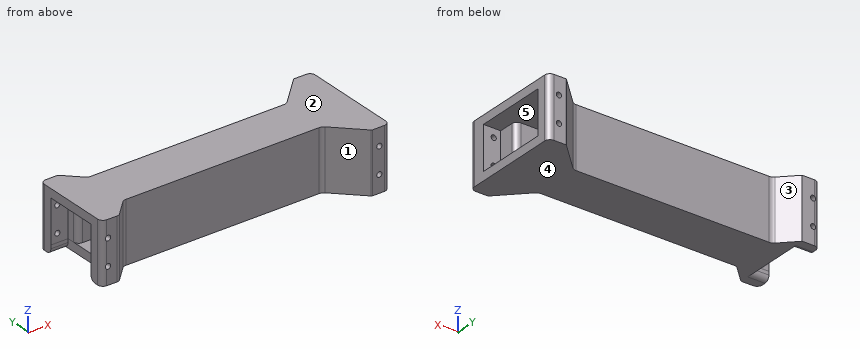
```python
from build123d import *

# Parameters (mm, degrees)
EXTRUDE_1_DEPTH     = 35
SKETCH_2_W          = 25
SKETCH_2_H          = 17
CUT_EXTRUDE_1_DEPTH = 173.018757571
SKETCH_4_W          = 25
SKETCH_4_H          = 13.5
SKETCH_4_H_2        = 11.5
CUT_EXTRUDE_2_DEPTH = 10
SKETCH_7_W          = 25
SKETCH_7_H          = 7
SKETCH_7_H_2        = 6.852029594
CUT_EXTRUDE_5_DEPTH = 10
FILLET_1_R          = 3
SKETCH_9_R          = 1.5
CUT_EXTRUDE_6_DEPTH = 270.810917265
CUT_EXTRUDE_8_DEPTH = 10
FILLET_3_R          = 3


with BuildPart() as part:
    # 草图1 → 凸台-拉伸1 (new body)
    with BuildSketch(Plane.XY):
        with BuildLine():
            Line((107.965790756, 7.914761882), (98.213694846, 7.766808503))
            Line((98.213694846, 7.766808503), (98.92442601, -39.079829993))
            Line((98.92442601, -39.079829993), (108.678766587, -39.079829993))
            ThreePointArc((108.678766587, -39.079829993), (108.959768197, -39.019490003), (109.19628872, -38.856208462))
            Line((109.19628872, -38.856208462), (117.753296763, -30.035556214))
            ThreePointArc((117.753296763, -30.035556214), (118.95311021, -29.207267035), (120.378565842, -28.901176343))
            Line((120.378565842, -28.901176343), (232.012858889, -27.207522891))
            ThreePointArc((232.012858889, -27.207522891), (233.446944009, -27.470230219), (234.671332156, -28.261740759))
            Line((234.671332156, -28.261740759), (250.089839512, -43.21939783))
            ThreePointArc((250.089839512, -43.21939783), (250.331204472, -43.375429159), (250.613907223, -43.427216939))
            Line((250.613907223, -43.427216939), (260.551832391, -43.276444261))
            Line((260.551832391, -43.276444261), (259.64165048, 16.716651749))
            Line((259.64165048, 16.716651749), (249.703725312, 16.565879071))
            ThreePointArc((249.703725312, 16.565879071), (249.422723701, 16.505539082), (249.186203178, 16.34225754))
            Line((249.186203178, 16.34225754), (234.228546108, 0.923750185))
            ThreePointArc((234.228546108, 0.923750185), (233.028732661, 0.095461006), (231.603277029, -0.210629686))
            Line((231.603277029, -0.210629686), (119.968983982, -1.904283139))
            ThreePointArc((119.968983982, -1.904283139), (118.534898862, -1.64157581), (117.310510715, -0.85006527))
            Line((117.310510715, -0.85006527), (108.489858467, 7.706942773))
            ThreePointArc((108.489858467, 7.706942773), (108.248493507, 7.862974102), (107.965790756, 7.914761882))
        make_face()
    extrude(amount=-EXTRUDE_1_DEPTH)

    # 草图2 → 切除-拉伸1 (cut, through all)
    with BuildSketch(Plane(origin=(259.835459196, 3.942079181, 0), x_dir=(0, 0, -1), z_dir=(0.999884933503295, 0.01516969851748372, 0))):
        with Locations((17.5, -17.223957338)):
            Rectangle(SKETCH_2_W, SKETCH_2_H)
    extrude(amount=-CUT_EXTRUDE_1_DEPTH, mode=Mode.SUBTRACT)

    # 草图4 → 切除-拉伸2 (cut)
    with BuildSketch(Plane(origin=(259.835459196, 3.942079181, 0), x_dir=(0, 0, -1), z_dir=(0.999884933503295, 0.01516969851748372, 0))):
        with Locations((17.5, -1.973957338)):
            Rectangle(SKETCH_4_W, SKETCH_4_H)
        with Locations((17.5, -31.473957338)):
            Rectangle(SKETCH_4_W, SKETCH_4_H_2)
    extrude(amount=-CUT_EXTRUDE_2_DEPTH, mode=Mode.SUBTRACT)

    # 草图7 → 切除-拉伸5 (cut)
    with BuildSketch(Plane(origin=(98.308900521, 1.491488003, 0), x_dir=(0, 0, 1), z_dir=(-0.9998849335032951, -0.015169698517482276, 0))):
        with Locations((-17.5, -5.223957338)):
            Rectangle(SKETCH_7_W, SKETCH_7_H)
        with Locations((-17.5, -29.149972135)):
            Rectangle(SKETCH_7_W, SKETCH_7_H_2)
    extrude(amount=-CUT_EXTRUDE_5_DEPTH, mode=Mode.SUBTRACT)

    # 圆角1
    # the kernel refuses this fillet: 3 mm, written as the material it takes off along each edge
    with BuildSketch(Plane(origin=(250.226834538, -21.930615176, -30), x_dir=(0.01516969851748703, -0.9998849335032949, 0), z_dir=(0, 0, 1)), Plane(origin=(249.968949663, -4.932571306, -5), x_dir=(-0.015169698517477554, 0.999884933503295, 0), z_dir=(0, 0, -1))) as fillet_1_piece_1:
        with BuildLine():
            CenterArc((FILLET_1_R, -FILLET_1_R), FILLET_1_R, 90, 90)
            Line((0, -FILLET_1_R), (0, 0))
            Line((0, 0), (FILLET_1_R, 0))
        make_face()
    extrude(amount=25, mode=Mode.SUBTRACT)
    with BuildSketch(Plane(origin=(98.92442601, -39.079829993, 7.387077266), x_dir=(1, 0, 0), z_dir=(0, 0, -1))) as fillet_1_piece_2:
        with BuildLine():
            CenterArc((FILLET_1_R * 0.984943635496, -FILLET_1_R), FILLET_1_R, 90, 89.13080696)
            Line((-FILLET_1_R * 0.0149412980072, -FILLET_1_R * 0.984830301483), (0, 0))
            Line((0, 0), (FILLET_1_R * 0.984943635496, 0))
        make_face()
    extrude(amount=49.774154532, mode=Mode.SUBTRACT)
    with BuildSketch(Plane(origin=(108.678766587, -39.079829993, 3.735844088), x_dir=(0.7926292381316349, 0.6097039370537671, 0), z_dir=(0, 0, -1))) as fillet_1_piece_3:
        with BuildLine():
            CenterArc((1.061212336, -2.968569096), FILLET_1_R, 81.698905724, 45.86919304)
            Line((-0.767899475, -0.590681381), (-0.950810656, -0.35289261))
            Line((-0.950810656, -0.35289261), (-0.182911181, 0.237788771))
            Line((-0.182911181, 0.237788771), (-0.17928295, 0.240536117))
            ThreePointArc((-0.17928295, 0.240536117), (0.589858632, 0.435143228), (1.537650165, 0.29685691))
            Line((1.537650165, 0.29685691), (1.494337635, 0))
        make_face()
    extrude(amount=42.471688176, mode=Mode.SUBTRACT)
    with BuildSketch(Plane(origin=(260.551832391, -43.276444261, 7.5), x_dir=(-0.015169698517487012, 0.9998849335032949, 0), z_dir=(0, 0, -1)), Plane(origin=(98.213694846, 7.766808503, 7.5), x_dir=(0.015169698517482278, -0.999884933503295, 0), z_dir=(0, 0, -1))) as fillet_1_piece_4:
        with BuildLine():
            CenterArc((FILLET_1_R, -FILLET_1_R), FILLET_1_R, 90, 90)
            Line((0, -FILLET_1_R), (0, 0))
            Line((0, 0), (FILLET_1_R, 0))
        make_face()
    extrude(amount=50, mode=Mode.SUBTRACT)
    with BuildSketch(Plane(origin=(259.64165048, 16.716651749, 7.5), x_dir=(0.015169698517487083, -0.9998849335032949, 0), z_dir=(0, 0, -1))) as fillet_1_piece_5:
        with BuildLine():
            CenterArc((FILLET_1_R, FILLET_1_R), FILLET_1_R, 180, 90)
            Line((0, FILLET_1_R), (0, 0))
            Line((0, 0), (FILLET_1_R, 0))
        make_face()
    extrude(amount=50, mode=Mode.SUBTRACT)
    with BuildSketch(Plane(origin=(108.440089659, -7.079768515, -30), x_dir=(0.9998849335032949, 0.015169698517490995, 0), z_dir=(0, 0, 1)), Plane(origin=(108.697974533, -24.077812384, -5), x_dir=(0.9998849335032949, 0.015169698517490636, 0), z_dir=(0, 0, -1))) as fillet_1_piece_6:
        with BuildLine():
            CenterArc((FILLET_1_R, FILLET_1_R), FILLET_1_R, 180, 90)
            Line((0, FILLET_1_R), (0, 0))
            Line((0, 0), (FILLET_1_R, 0))
        make_face()
    extrude(amount=25, mode=Mode.SUBTRACT)

    # 草图9 → 切除-拉伸6 (cut, through all)
    with BuildSketch(Plane(origin=(0.716373196, -47.218523443, 0), x_dir=(0.999884933503295, 0.015169698517483048, 0), z_dir=(0.015169698517483048, -0.999884933503295, 0))):
        with Locations((253.92629217, -25)):
            Circle(SKETCH_9_R)
        with Locations((253.92629217, -10)):
            Circle(SKETCH_9_R)
        with Locations((102.073432063, -10)):
            Circle(SKETCH_9_R)
        with Locations((102.073432063, -25)):
            Circle(SKETCH_9_R)
    extrude(amount=-CUT_EXTRUDE_6_DEPTH, mode=Mode.SUBTRACT)

    # 草图11 → 切除-拉伸8 (cut)
    with BuildSketch(Plane(origin=(0, 0, -35), x_dir=(-1, 0, 0), z_dir=(0, 0, -1))):
        Polygon((-98.335052434, -0.232270965), (-98.803068421, -31.080750525), (-108.801917756, -30.929053539), (-108.333901769, -0.08057398), align=None)
    extrude(amount=-CUT_EXTRUDE_8_DEPTH, mode=Mode.SUBTRACT)

    # 圆角3
    fillet_3_edges = [part.edges().sort_by_distance(p)[0] for p in [
        (103.334477101, -0.156422473, -35),
        (103.802493089, -31.004902032, -35),
    ]]
    fillet(fillet_3_edges, radius=FILLET_3_R)


solid = part.part
```
The listing builds one solid part. Answer for the finished solid, in the listing's coordinates (mm). Face numbers are marked on the shaded views. A direction names the side the tool comes from. Coordinates: 2 decimals unless noted, no trailing zeros. Write each loop counter-clockwise with the first axis right and the second up, starting at its lowest first coordinate (ties: lowest second). Pieces come first, ordered by that corner, then holes. Notation, with made-up numbers: (30, 79) - (83, 79) arc R27 ccw to (83, 104) - close; hole circle Ø5 at (16.25, -32.5). An arc over 180 degrees is marked (long way). Return JSON: item names as keys, results as strings. Group by question number.
Q1. The part is cut by section C-C on y = 11.5. State how many separate pieces and enclosed holes the cut face has, and give its area (3 significant figures).
Q2. The part is cut by section A-A on y = -18. Write down the section's boundary in (x, z), and give its area (3 significant figures).
Q3. Find the intervals of material crossed by line 1 along Z through (x, y) = (133, -22.5); line 2 along Y through (x, z) = (253.5, -3.5); line 3 along Y through (x, z) = (107, -16), in increasing order. Write a range as [from, to].
Q4. The part is cut by section B-B on x = 142. Write down the section's boundary in (y, z).
Q5. Which of the six approach directions +Z, -Z, +X, -X, +Y, -Y give full straight-line access (tool end or side, diameter ignored) to the marked faces 1 and 2?
Q6. Flat-ended cylindrical pins translate along their axes: pin 1 Ø5 at (x, z) = (152, -7) entering from -Y; pin 2 Ø21 at (x, y) = (176.5, -5.5) entering from +Z; pin 3 Ø1.7 at (x, z) = (103.5, -20) entering from -Y; pin 4 Ø2 at (x, z) = (192.5, -26.5) entering from +Y. Find the tip coordinate at first contact, or state that the pin passes through.
Q7. For a pull along Y with two mould halves and no side action, classify the marked faces 3, 4 and 5 as +Y half, -Y half, draft (parallel to the pull), parting line (faces both ways), or undercut.
Evaluation:
{
 "1": {"separate pieces": "1", "enclosed holes": "2", "area": "519 mm2"},
 "2": {"outline": "(98.6, -5) - (260.17, -5) - (260.17, 0) - (98.6, 0) - close; (108.61, -35) - (260.17, -35) - (260.17, -30) - (108.61, -30) - close", "area": "1,570 mm2"},
 "3": {"line 1": "z = [-35, -30], [-5, 0]", "line 2": "y = [-43.38, 16.62]", "line 3": "y = [-39.08, -30.96], [-0.1, 7.9]"},
 "4": {"outline": "(-28.57, -35) - (-1.57, -35) - (-1.57, 0) - (-28.57, 0) - close; hole (-23.57, -30) - (-6.57, -30) - (-6.57, -5) - (-23.57, -5) - close"},
 "5": {"face 1": "+Z, -Z, -Y", "face 2": "+Z, +X, -X, +Y, -Y"},
 "6": {"pin 1": "stops at y = -28.46", "pin 2": "stops at z = 0", "pin 3": "stops at y = -39.08", "pin 4": "stops at y = -0.79"},
 "7": {"face 3": "+Y half", "face 4": "draft", "face 5": "undercut"}
}
